```python
from build123d import *

# Parameters (mm, degrees)
F0_R        = 1.27
F0_R_2      = 3.96875
F1_DEPTH    = 6.35
F2_R        = 6.477
F2_R_2      = 1.27
F3_DEPTH    = 6.35
F4_S5_R     = 6.477
F4_T6_DEPTH = 13
F5_W        = 12.7
F5_H        = 3.81
F6_DEPTH    = 14.9999954
F8_DEPTH    = 25.4
F9_W        = 12.7
F9_H        = 3.81
F10_DEPTH   = 14.9999954
F12_DEPTH   = 25.4
F13_W       = 3.175
F13_H       = 12.7
F14_DEPTH   = 14.9999954
F16_DEPTH   = 25.4


# Not quite as in the source:
# - a fillet or chamfer that OpenCascade refuses, or shapes differently, is made with other operations: its cross-section is extruded or revolved along the edge and cut away or added
# - after a boolean that leaves OpenCascade's solid faulty, fix() repairs it
# - ends of sketch curves that miss each other by under 0.0002 mm in the source are joined


with BuildPart() as f1:
    # F0 (on Front) → F1 (new body)
    with BuildSketch(Plane.XZ):
        Polygon((-7.493, 0.1328983575), (0, 0.1328983575), (7.493, 0.1328983575), (22.2194990303, 0.1328983575), (22.2194990303, 19.5094533027), (14.8570176459, 25.8122983575), (7.7658264293, 31.8828983575), (7.7658264293, 38.2328983575), (-7.7713273633, 38.2328983575), (-7.7713273633, 31.8828983575), (-14.8625185798, 25.8122983575), (-22.2249999642, 19.5094533027), (-22.2249999642, 4.5234533027), (-22.2249999642, 0.1328983575), align=None)
        with Locations((-3.175, 36.0046029091)):
            Circle(F0_R, mode=Mode.SUBTRACT)
        with BuildLine():
            ThreePointArc((-1.6471995105, 13.7654938087), (-14.0416307026, 9.056743723), (-13.4701421127, 22.3031640975))
            Line((-13.4701421127, 22.3031640975), (-7.8430329322, 27.1203983575))
            Line((-7.8430329322, 27.1203983575), (-3.175, 27.1203983575))
            Line((-3.175, 27.1203983575), (-3.175, 30.2953983575))
            Line((-3.175, 30.2953983575), (-3.175, 33.4703983575))
            Line((-3.175, 33.4703983575), (3.175, 33.4703983575))
            Line((3.175, 33.4703983575), (3.175, 30.2953983575))
            Line((3.175, 30.2953983575), (3.175, 27.1203983575))
            Line((3.175, 27.1203983575), (7.8375319983, 27.1203983575))
            Line((7.8375319983, 27.1203983575), (13.4701421127, 22.3031640975))
            ThreePointArc((13.4701421127, 22.3031640975), (16.2995077669, 19.40684068), (17.3322006389, 15.4917998403))
            ThreePointArc((17.3322006389, 15.4917998403), (10.2711150187, 7.6028326022), (1.6507381924, 13.7496885133))
            ThreePointArc((1.6507381924, 13.7496885133), (0.0063534061, 14.7141035739), (-1.6471995105, 13.7654938087))
        make_face(mode=Mode.SUBTRACT)
        with Locations((3.175, 36.0046029091)):
            Circle(F0_R, mode=Mode.SUBTRACT)
        Polygon((14.8570176459, 25.8122983575), (22.2194990303, 19.5094533027), (22.2194990303, 25.8122983575), (17.4187807526, 25.8122983575), align=None)
        Polygon((-22.2249999642, 25.8122983575), (-22.2249999642, 19.5094533027), (-14.8625185798, 25.8122983575), (-17.4242816865, 25.8122983575), align=None)
        with BuildLine():
            ThreePointArc((13.4519986436, 22.3139871107), (4.7326542757, 21.9159130054), (1.6507381924, 13.7496885133))
            ThreePointArc((1.6507381924, 13.7496885133), (10.2711150187, 7.6028326022), (17.3322006389, 15.4917998403))
            ThreePointArc((17.3322006389, 15.4917998403), (16.2995077669, 19.40684068), (13.4701421127, 22.3031640975))
            ThreePointArc((13.4701421127, 22.3031640975), (13.461073979, 22.3085816404), (13.4519986436, 22.3139871107))
        make_face()
        with BuildLine():
            ThreePointArc((-1.4572006389, 15.4917998403), (-5.4796598384, 22.3966069904), (-13.4701421898, 22.3031640514))
            ThreePointArc((-13.4701421127, 22.3031640975), (-14.0416307026, 9.056743723), (-1.6471995105, 13.7654938087))
            ThreePointArc((-1.6471995105, 13.7654938087), (-1.5048433381, 14.6234346974), (-1.4572006389, 15.4917998403))
        make_face()
        with BuildLine():
            Line((-7.8430329322, 27.1203983575), (-13.4701422669, 22.3031640053))
            ThreePointArc((-13.4701421898, 22.3031640514), (-5.4796598384, 22.3966069904), (-1.4572006389, 15.4917998403))
            ThreePointArc((-1.4572006389, 15.4917998403), (-1.5048433381, 14.6234346974), (-1.6471995105, 13.7654938087))
            ThreePointArc((-1.6471995105, 13.7654938087), (0.0063534061, 14.7141035739), (1.6507381924, 13.7496885133))
            ThreePointArc((1.6507381924, 13.7496885133), (4.7326542757, 21.9159130054), (13.4519986436, 22.3139871107))
            Line((13.4519986436, 22.3139871107), (7.8375319983, 27.1203983575))
            Line((7.8375319983, 27.1203983575), (3.175, 27.1203983575))
            Line((3.175, 27.1203983575), (3.175, 30.2953983575))
            Line((3.175, 30.2953983575), (3.175, 33.4703983575))
            Line((3.175, 33.4703983575), (-3.175, 33.4703983575))
            Line((-3.175, 33.4703983575), (-3.175, 30.2953983575))
            Line((-3.175, 30.2953983575), (-3.175, 27.1203983575))
            Line((-3.175, 27.1203983575), (-7.8430329322, 27.1203983575))
        make_face()
        with Locations((0, 23.0759866536)):
            Circle(F0_R_2, mode=Mode.SUBTRACT)
    extrude(amount=F1_DEPTH)

    # F2 (on face) → F3 (join)
    with BuildSketch(Plane(origin=(0, 0, 0), x_dir=(-1, 0, 0), z_dir=(0, 1, 0))):
        Polygon((-22.2194990303, 25.8122983575), (-22.2194990303, 0.1328983575), (22.2249999642, 0.1328983575), (22.2249999642, 25.8122983575), (14.8625185798, 25.8122983575), (7.7713273633, 31.8828983575), (7.7713273633, 38.2328983575), (-7.7658264293, 38.2328983575), (-7.7658264293, 31.8828983575), (-14.8570176459, 25.8122983575), align=None)
        with Locations((0, 23.0759866536)):
            Circle(F2_R, mode=Mode.SUBTRACT)
        with Locations((-3.175, 36.0046029091)):
            Circle(F2_R_2, mode=Mode.SUBTRACT)
        with Locations((3.175, 36.0046029091)):
            Circle(F2_R_2, mode=Mode.SUBTRACT)
    extrude(amount=F3_DEPTH)

    # F4: chamfer of 3.81 x 6.5991135768 on 1 edges, made by hand


with BuildPart() as f4_tool2:
    # F4_s3 → F4_t4 (revolve)
    with BuildSketch(Plane.XY.offset(23.0759866536)):
        Polygon((7.77875, 0), (3.96875, -6.5991135768), (3.96875, 0), align=None)
    revolve(axis=Axis((0, 0, 23.0759866536), (0, -1, 0)))

    # F4_s5 → F4_t6 (intersect, symmetric)
    with BuildSketch(Plane.XZ.offset(3.3)):
        with Locations((0, 23.0759866536)):
            Circle(F4_S5_R)
    extrude(amount=F4_T6_DEPTH, both=True, mode=Mode.INTERSECT)


with BuildPart() as f1_1:
    add(f1.part)

    # F4_t1: cut F4_tool2
    add(f4_tool2.part, mode=Mode.SUBTRACT)

    # F5 (on face) → F6 (join)
    with BuildSketch(Plane(origin=(-22.2249999642, 0, 0), x_dir=(0, -1, 0), z_dir=(-1, 0, 0))):
        with Locations((0, 23.9072983575)):
            Rectangle(F5_W, F5_H)
    extrude(amount=F6_DEPTH)

    # F7 (on face) → F8 (cut)
    with BuildSketch(Plane(origin=(0, 0, 22.0022983575), x_dir=(1, 0, 0), z_dir=(0, 0, -1))):
        with BuildLine():
            ThreePointArc((-28.7557423483, 0.8206364192), (-30.5456340834, 0.969255316), (-30.6942529802, -0.8206364192))
            Line((-30.6942529802, -0.8206364192), (-28.7557423483, 0.8206364192))
        make_face()
        with BuildLine():
            Line((-28.7557423483, 0.8206364192), (-30.6942529802, -0.8206364192))
            ThreePointArc((-30.6942529802, -0.8206364192), (-29.2879932313, -1.1924458586), (-28.4549976642, 0))
            ThreePointArc((-28.4549976642, 0), (-28.5325518057, 0.4370044329), (-28.7557423483, 0.8206364192))
        make_face()
    extrude(amount=-F8_DEPTH, mode=Mode.SUBTRACT)

    # F9 (on face) → F10 (join)
    with BuildSketch(Plane.YZ.offset(22.2194990303)):
        with Locations((0, 23.9072983575)):
            Rectangle(F9_W, F9_H)
    extrude(amount=F10_DEPTH)

    # F11 (on face) → F12 (cut)
    with BuildSketch(Plane(origin=(0, 0, 22.0022983575), x_dir=(1, 0, 0), z_dir=(0, 0, -1))):
        with BuildLine():
            ThreePointArc((30.9894967303, 0), (30.9119425889, 0.4370044329), (30.6887520463, 0.8206364192))
            Line((30.6887520463, 0.8206364192), (28.7502414143, -0.8206364192))
            ThreePointArc((28.7502414143, -0.8206364192), (30.1565011632, -1.1924458586), (30.9894967303, 0))
        make_face()
        with BuildLine():
            Line((28.7502414143, -0.8206364192), (30.6887520463, 0.8206364192))
            ThreePointArc((30.6887520463, 0.8206364192), (28.8988603111, 0.969255316), (28.7502414143, -0.8206364192))
        make_face()
    extrude(amount=-F12_DEPTH, mode=Mode.SUBTRACT)

    # F13 (on face) → F14 (join)
    with BuildSketch(Plane(origin=(0, 0, 0.1328983575), x_dir=(1, 0, 0), z_dir=(0, 0, -1))):
        with Locations((9.0874977, 0)):
            Rectangle(F13_W, F13_H)
        with Locations((-9.0874977, 0)):
            Rectangle(F13_W, F13_H)
    extrude(amount=F14_DEPTH)

    add(f1_1.part.fix(), mode=Mode.REPLACE)

    # F15 (on face) → F16 (cut)
    with BuildSketch(Plane.YZ.offset(10.6749977)):
        with BuildLine():
            ThreePointArc((1.27, -7.3670993425), (0.5341777549, -6.2149039918), (-0.8206364192, -6.3978440265))
            Line((-0.8206364192, -6.3978440265), (0.8206364192, -8.3363546585))
            ThreePointArc((0.8206364192, -8.3363546585), (1.1521953507, -7.9012770974), (1.27, -7.3670993425))
        make_face()
        with BuildLine():
            Line((0.8206364192, -8.3363546585), (-0.8206364192, -6.3978440265))
            ThreePointArc((-0.8206364192, -6.3978440265), (-0.969255316, -8.1877357617), (0.8206364192, -8.3363546585))
        make_face()
    extrude(amount=-F16_DEPTH, mode=Mode.SUBTRACT)


solid = f1_1.part
```
CAD build for the part. Positions are in the model's coordinates, mm. A direction names the side the tool comes from. Coordinates: 2 decimals unless noted, no trailing zeros. Order: outer loops, then holes, each group sorted by start corner. A loop starts at its lowest first (then second) coordinate and runs counter-clockwise, first axis right, second up. Notation, with made-up numbers: M 18.5,-18 L 37.5,-18 A28 cw 37.5,8 Z; hole C 36.5,33 d8. An arc over 180 degrees is marked long. Write each question's results on one line, items separated by ' | '. Start each with the question number.
Q1. Drill centre lines: probe 1 along X at (y, z) = (3.5, -5.5) (3 decimals); probe 2 along Z at (x, y) = (-30, -4.75); probe 3 along X at (y, z) = (-4.5, 14.5) (1 decimal). Where is each one in solid material? Low to high. Write a range as from..to.
Q2. Pull direction Z, two halves, no side cores. Call faces 1 (the flat face through (26, 0, 25.812)), 2 (the conical face through (-3.35, -6.15, 20.5)), 3 (the flat face through (22.219, 0, 11)): +Z half, -Z half, draft (parallel to the pull), parting line (faces both ways), or undercut.
Q3. Cut at D-D (y = -3.25). Count the separate pieces of the cut face and the enclosed holes in it, then the cut area to 3 significant figures.
Q4. Cut at A-A (x = 0). List the corners of the cut face in (y, z).
Q5. Which spindle directions (+Z, -Z, +X, -X, +Y, -Y) get a long thin tool onto all of the face, cutting with end or side? Do faces 4 (the flat face through (-22.225, 0, 11)), 5 (the flat face through (30, -2, 22.002)), 6 (the flat face through (-26, 0, 25.812)). Say none if no direction does.
Q6. Cut at B-B (y = 4). List the corners of the cut face in (x, z) (1 decimal), then the cut area to 3 significant figures.
Q7. Flat gauge pins, fed straight in: P1, Ø3, axis at y = 3, z = 34, coming from the -X side; P2, Ø6, axis at y = -2.5, z = 32.5, coming from the +X side; P3, Ø6.5, axis at x = -26.5, y = 1.5, coming from the +Z side. Where does each tip first touch, or does it go through?
Found:
1) probe 1: -10.675..-7.5, 7.5..10.675 | probe 2: 22..25.81 | probe 3: -22.2..22.2
2) face 1: +Z half | face 2: undercut | face 3: draft
3) separate pieces: 1 | enclosed holes: 4 | area: 1,470 mm²
4) outline: M -6.35,0.13 L 6.35,0.13 L 6.35,16.6 L -2.25,16.6 L -6.35,18.96 Z; M -6.35,27.19 L -2.25,29.55 L 6.35,29.55 L 6.35,38.23 L -6.35,38.23 Z
5) face 4: -Z, -X, +Y, -Y | face 5: -Z, +X, +Y, -Y | face 6: +Z, -X, +Y, -Y
6) outline: M -37.2,22 L -22.2,22 L -22.2,0.1 L -10.7,0.1 L -10.7,-14.9 L -7.5,-14.9 L -7.5,0.1 L 7.5,0.1 L 7.5,-14.9 L 10.7,-14.9 L 10.7,0.1 L 22.2,0.1 L 22.2,22 L 37.2,22 L 37.2,25.8 L 14.9,25.8 L 7.8,31.9 L 7.8,38.2 L -7.8,38.2 L -7.8,31.9 L -14.9,25.8 L -37.2,25.8 Z; hole C 0,23.1 d13; hole C -3.2,36 d2.5; hole C 3.2,36 d2.5 | area: 1,440 mm²
7) P1: x = -7.77 | P2: x = 10.55 | P3: z = 25.81
